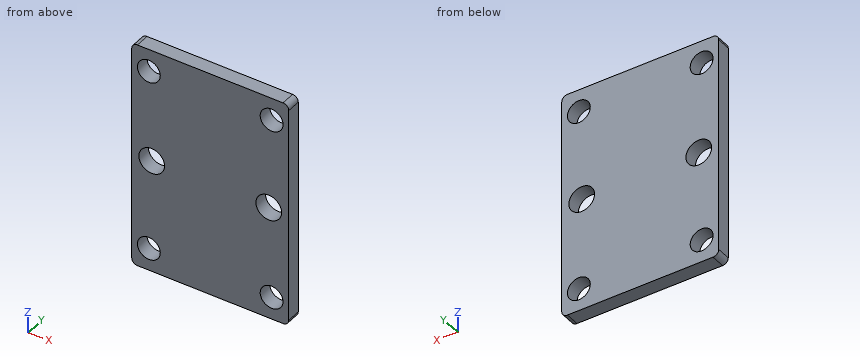
from build123d import *

# Parameters (mm, degrees)
SALIENTE_EXTRUIR1_DEPTH = 5
CROQUIS2_R              = 4.5
CROQUIS2_R_2            = 4
CORTAR_EXTRUIR1_DEPTH   = 10


with BuildPart() as part:
    # Croquis1 → Saliente-Extruir1 (new body)
    with BuildSketch(Plane(origin=(0, 0, 0), x_dir=(1, 0, 0), z_dir=(0, 1, 0))):
        with BuildLine():
            Line((-27.5, -38), (-27.5, 38))
            ThreePointArc((-27.5, 38), (-26.914213562, 39.414213562), (-25.5, 40))
            Line((-25.5, 40), (25.5, 40))
            ThreePointArc((25.5, 40), (26.914213562, 39.414213562), (27.5, 38))
            Line((27.5, 38), (27.5, -38))
            ThreePointArc((27.5, -38), (26.914213562, -39.414213562), (25.5, -40))
            Line((25.5, -40), (-25.5, -40))
            ThreePointArc((-25.5, -40), (-26.914213562, -39.414213562), (-27.5, -38))
        make_face()
    extrude(amount=SALIENTE_EXTRUIR1_DEPTH)

    # Croquis2 → Cortar-Extruir1 (cut)
    with BuildSketch(Plane(origin=(0, 5, 0), x_dir=(1, 0, 0), z_dir=(0, 1, 0))):
        with Locations(Location((-20.5, 0, 0), (0, 0, 270))):
            Circle(CROQUIS2_R)
        with Locations(Location((20.5, 0, 0), (0, 0, 270))):
            Circle(CROQUIS2_R)
        with Locations(Location((-21.5, 32.1, 0), (0, 0, 270))):
            Circle(CROQUIS2_R_2)
        with Locations(Location((-21.5, -32.1, 0), (0, 0, 270))):
            Circle(CROQUIS2_R_2)
        with Locations(Location((21.5, 32.1, 0), (0, 0, 270))):
            Circle(CROQUIS2_R_2)
        with Locations(Location((21.5, -32.1, 0), (0, 0, 270))):
            Circle(CROQUIS2_R_2)
    extrude(amount=-CORTAR_EXTRUIR1_DEPTH, mode=Mode.SUBTRACT)


solid = part.part
Geometry: final body of the model. Coordinates: model frame, mm. Coordinates: 2 decimals unless noted, no trailing zeros. Loops run counter-clockwise (first coordinate to the right, second up) from the corner with the lowest first, then second, coordinate; pieces in that order, holes last. Notation, with made-up numbers: (55, -3) - (76, -3) arc R21 ccw to (76, 25) - close; hole circle Ø6 at (70, 34.5). An arc over 180 degrees is marked (long way). One line per question, with ' | ' between items. Start each with the question number.
(1) Cut plane C-C on x = -19.5. Output: boundary loops of the cut face in (y, z).
(2) Cut plane B-B on z = 0. Output: boundary loops of the cut face in (x, y).
(3) Cut plane A-A on y = 2.95. Output: boundary loops of the cut face in (x, z), and give its area (3 significant figures).
(4) Ray query, L1, parallel to X at y = 1.9, z = -32.1; L2, parallel to X at y = 1.65, z = 0; L3, parallel to Z at x = 18.5, y = 1.4. Return the intervals inside material, ascending. Write a range as from..to.
(5) Cut plane D-D on z = 31. Output: boundary loops of the cut face in (x, y).
Here are the results:
1) outline: (0, -40) - (5, -40) - (5, -35.56) - (0, -35.56) - close; (0, -28.64) - (5, -28.64) - (5, -4.39) - (0, -4.39) - close; (0, 4.39) - (5, 4.39) - (5, 28.64) - (0, 28.64) - close; (0, 35.56) - (5, 35.56) - (5, 40) - (0, 40) - close
2) outline: (-27.5, 0) - (-25, 0) - (-25, 5) - (-27.5, 5) - close; (-16, 0) - (16, 0) - (16, 5) - (-16, 5) - close; (25, 0) - (27.5, 0) - (27.5, 5) - (25, 5) - close
3) outline: (-27.5, -38) arc R2 ccw to (-25.5, -40) - (25.5, -40) arc R2 ccw to (27.5, -38) - (27.5, 38) arc R2 ccw to (25.5, 40) - (-25.5, 40) arc R2 ccw to (-27.5, 38) - close; hole circle Ø8 at (-21.5, -32.1); hole circle Ø8 at (-21.5, 32.1); hole circle Ø9 at (-20.5, 0); hole circle Ø9 at (20.5, 0); hole circle Ø8 at (21.5, -32.1); hole circle Ø8 at (21.5, 32.1) | area: 4,070 mm²
4) L1: -27.5..-25.5, -17.5..17.5, 25.5..27.5 | L2: -27.5..-25, -16..16, 25..27.5 | L3: -40..-34.75, -29.45..-4.03, 4.03..29.45, 34.75..40
5) outline: (-27.5, 0) - (-25.35, 0) - (-25.35, 5) - (-27.5, 5) - close; (-17.65, 0) - (17.65, 0) - (17.65, 5) - (-17.65, 5) - close; (25.35, 0) - (27.5, 0) - (27.5, 5) - (25.35, 5) - close
